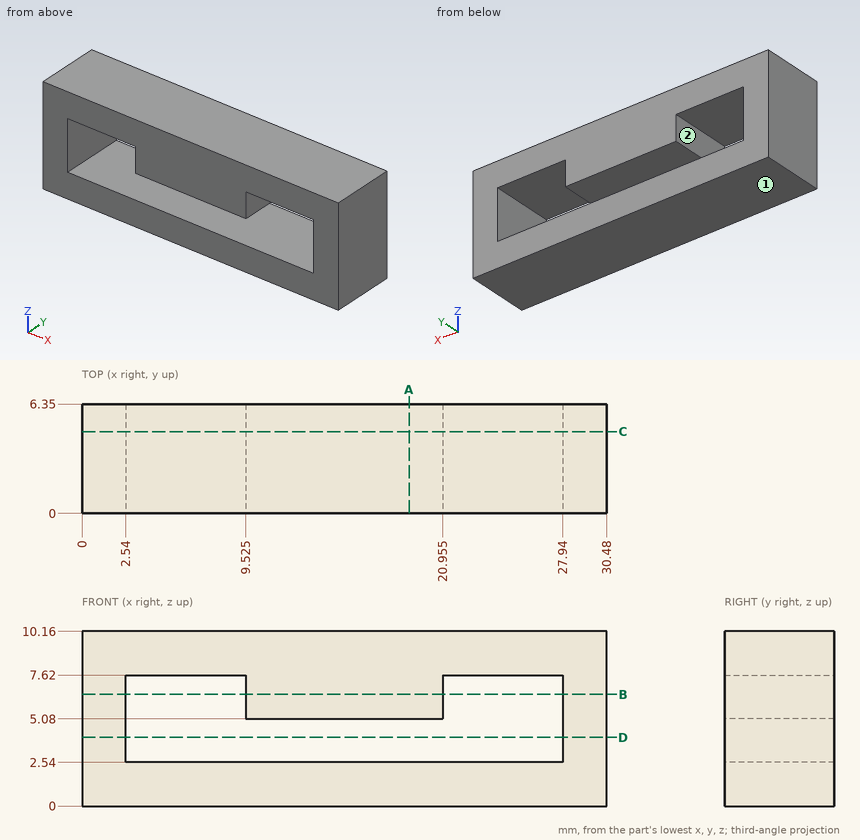
Here's the drawing with two shaded views (mm, measured from the low corner). I have some questions. A direction names the side the tool comes from. Give positions to 0.01 mm unless a question says otherwise; leave off trailing zeros. Order: outer loops, then holes, each group sorted by start corner. A loop starts at its lowest first (then second) coordinate and runs counter-clockwise, first axis right, second up. Notation, with made-up numbers: (30, 59) -> (80, 59) arc R24 cw to (80, 73) -> close; hole circle Ø5 at (33.25, -29). An arc over 180 degrees is marked (long way). Use a Markdown table: item, result. Add a question column.
Item 1: Imagine slicing it at D-D on z = 4. Please give me the cut outline in (x, y).
Item 2: Imagine slicing it at A-A on x = 19. Please give me the cut outline in (y, z).
Item 3: Will this pin go through, and if not, where does the flat tip stop? pin 1 (3 mm diameter, centred on x = 7, y = 2.5, fed in from -Z).
Item 4: For the marked faces 1 and 2, which set-ups out of +Z, -Z, +X, -X, +Y, -Y let a thin tool reach every point of the face, with its end or its side?
Item 5: I need wall thicknesses on line 1 (Z direction, x = 10.5, y = 5.5); line 2 (X direction, y = 0.5, z = 6.5) (3 decimals); line 3 (Z direction, x = 24, y = 2). Which ranges of each line are inside material? Lowest first, please.
Item 6: Imagine slicing it at C-C on y = 4.75. Please give me the cut outline in (x, z) (3 decimals), plus the area to 3 significant figures.
Item 7: Imagine slicing it at B-B on z = 6.5. Please give me the cut outline in (x, y) (3 decimals), plus the area to 3 significant figures.
Data:
| question | item | result |
|---|---|---|
| 1 | outline | (0, 0) -> (2.54, 0) -> (2.54, 6.35) -> (0, 6.35) -> close; (27.94, 0) -> (30.48, 0) -> (30.48, 6.35) -> (27.94, 6.35) -> close |
| 2 | outline | (0, 0) -> (6.35, 0) -> (6.35, 2.54) -> (0, 2.54) -> close; (0, 5.08) -> (6.35, 5.08) -> (6.35, 10.16) -> (0, 10.16) -> close |
| 3 | pin 1 | stops at z = 0 |
| 4 | face 1 | -Z, +X, -X, +Y, -Y |
| 4 | face 2 | +Y, -Y |
| 5 | line 1 | z = 0 to 2.54, 5.08 to 10.16 |
| 5 | line 2 | x = 0 to 2.54, 9.525 to 20.955, 27.94 to 30.48 |
| 5 | line 3 | z = 0 to 2.54, 7.62 to 10.16 |
| 6 | outline | (0, 0) -> (30.48, 0) -> (30.48, 10.16) -> (0, 10.16) -> close; hole (2.54, 2.54) -> (27.94, 2.54) -> (27.94, 7.62) -> (20.955, 7.62) -> (20.955, 5.08) -> (9.525, 5.08) -> (9.525, 7.62) -> (2.54, 7.62) -> close |
| 6 | area | 210 mm² |
| 7 | outline | (0, 0) -> (2.54, 0) -> (2.54, 6.35) -> (0, 6.35) -> close; (9.525, 0) -> (20.955, 0) -> (20.955, 6.35) -> (9.525, 6.35) -> close; (27.94, 0) -> (30.48, 0) -> (30.48, 6.35) -> (27.94, 6.35) -> close |
| 7 | area | 105 mm² |
